Geometry check sheet. Reference: the model listing, model coordinates, mm. A direction names the side the tool comes from. Round coordinates to 2 decimals unless told otherwise and drop trailing zeros. Order: outer loops, then holes, each group sorted by start corner. A loop starts at its lowest first (then second) coordinate and runs counter-clockwise, first axis right, second up. Notation, with made-up numbers: (66.5, 88) - (123.5, 88) arc R15 ccw to (123.5, 102) - close; hole circle Ø4 at (41, 20.5). An arc over 180 degrees is marked (long way). Use a Markdown table: item, result. Add a question column.
(1) Thickness scan on line 1 along Y through (x, z) = (38.1, 0.6) (3 decimals); line 2 along Y through (x, z) = (19.05, 2); line 3 along X through (y, z) = (11.5, 1) (3 decimals). Record the ranges inside material, lowest first. Write a range as [from, to].
(2) Section check C-C on x = 38.1. Record the boundary of the cut face in (y, z) (3 decimals), then the cut area to 3 significant figures.
(3) Access from +Z, -Z, +X, -X, +Y, -Y to the whole of each face (thin tool, end or side, straight path). Record for faces 4 (the face through (-37, 11, 2.381)), 5 (the face through (-32.84, 12.03, 3.22)), 6 (the face through (-0.15, 12.39, 3.22)).
(4) Gauge pin test, flat end, axial feed: P1, Ø1, axis at x = -25.5, z = 5.5, coming from the +Y side. Record the tip position at first contact, or that the pin passes through.
(5) Mould release check, pull along X, two halves, no side actions. Record for faces 1 (the face through (34, 16.9, 3.2)), 2 (the face through (39, 11, 2.381)), 3 (the face through (20, 19.05, 3)): released by +X, released by -X, zero draft, split by the parting line, or undercut.
(6) Section check B-B on z = 1.5. Give the number of separate pieces and of enclosed holes in the cut face, then the cut area to 3 significant figures.
(7) Section check D-D on x = -38.1. Record the boundary of the cut face in (y, z), then the cut area to 3 significant figures.
(8) Section check A-A on x = 19.05. Record the boundary of the cut face in (y, z), then the cut area to 3 significant figures.
```python
from build123d import *

# Parameters (mm, degrees)
SKETCH1_W          = 88.9
SKETCH1_H          = 19.05
BASE_EXTRUDE_DEPTH = 6.35
CUT_EXTRUDE1_DEPTH = 49.775275499
CUT_EXTRUDE2_DEPTH = 49.775275499
CUT_EXTRUDE3_DEPTH = 49.775275499
CUT_EXTRUDE4_DEPTH = 49.775275499
CUT_EXTRUDE5_DEPTH = 49.775275499
FILLET1_R          = 3.175
HOLE1_D            = 7.14375
HOLE1_CBORE_D      = 10.31875
HOLE1_CBORE_DEPTH  = 3.96875
LPATTERN1_COUNT    = 2
LPATTERN1_PITCH    = 76.2
HOLE2_OUTLINE_R    = 1.5875
HOLE2_DEPTH        = 6.35
HOLE3_OUTLINE_R    = 1.5875
HOLE3_DEPTH        = 6.35
LPATTERN2_COUNT    = 2
LPATTERN2_PITCH    = 57.15


# Read off the part's stored shape, not the designer's step: Hole2, Hole3
with BuildPart() as part:
    # Sketch1 → Base-Extrude (new body)
    with BuildSketch(Plane.XY):
        with Locations((0, 9.525)):
            Rectangle(SKETCH1_W, SKETCH1_H)
    extrude(amount=BASE_EXTRUDE_DEPTH)

    # Sketch2 → Cut-Extrude1 (cut, through all)
    with BuildSketch(Plane.XY.offset(6.35)):
        Polygon((44.45, 14.2875), (25.4, 19.05), (44.45, 19.05), align=None)
    extrude(amount=-CUT_EXTRUDE1_DEPTH, mode=Mode.SUBTRACT)

    # Sketch3 → Cut-Extrude2 (cut, through all)
    with BuildSketch(Plane.XY.offset(6.35)):
        with BuildLine():
            Line((-136.365872597, 74.873193339), (-14.549677831, 19.05))
            ThreePointArc((-14.549677831, 19.05), (0, 15.875), (14.549677831, 19.05))
            Line((14.549677831, 19.05), (136.365872597, 74.873193339))
            Line((136.365872597, 74.873193339), (136.365872597, 342.868821823))
            Line((136.365872597, 342.868821823), (-136.365872597, 342.868821823))
            Line((-136.365872597, 342.868821823), (-136.365872597, 74.873193339))
        make_face()
    extrude(amount=-CUT_EXTRUDE2_DEPTH, mode=Mode.SUBTRACT)

    # Sketch4 → Cut-Extrude3 (cut, through all)
    with BuildSketch(Plane.XY.offset(6.35)):
        Polygon((-231.275885049, -20.742353447), (-44.45, 14.2875), (-19.05, 19.05), (167.775885049, 54.079853447), (97.716178156, 427.731623544), (-301.335591942, 352.909416651), align=None)
    extrude(amount=-CUT_EXTRUDE3_DEPTH, mode=Mode.SUBTRACT)

    # Sketch5 → Cut-Extrude4 (cut, through all)
    with BuildSketch(Plane.XY.offset(6.35)):
        Polygon((-36.984386732, 15.687302488), (-28.575, 8.262261056), (-28.575, 17.2640625), align=None)
    extrude(amount=-CUT_EXTRUDE4_DEPTH, mode=Mode.SUBTRACT)

    # Sketch6 → Cut-Extrude5 (cut, through all)
    with BuildSketch(Plane.XY.offset(6.35)):
        with BuildLine():
            ThreePointArc((-10.587110246, 13.878358811), (0, 12.3904375), (10.587110246, 13.878358811))
            ThreePointArc((10.587110246, 13.878358811), (14.75971189, 11.565447951), (12.446801031, 7.392846306))
            ThreePointArc((12.446801031, 7.392846306), (0, 5.6435625), (-12.446801031, 7.392846306))
            ThreePointArc((-12.446801031, 7.392846306), (-14.75971189, 11.565447951), (-10.587110246, 13.878358811))
        make_face()
    extrude(amount=-CUT_EXTRUDE5_DEPTH, mode=Mode.SUBTRACT)

    # Fillet1
    fillet1_edges = [part.edges().sort_by_distance(p)[0] for p in [
        (44.45, 14.2875, 3.175),
        (25.4, 19.05, 3.175),
        (-19.05, 19.05, 3.175),
        (-44.45, 14.2875, 3.175),
    ]]
    fillet(fillet1_edges, radius=FILLET1_R)

    # Hole1 (through all)
    with Locations(Plane.XY.offset(6.35)):
        with Locations((38.1, 7.14375)):
            hole1 = CounterBoreHole(HOLE1_D / 2, HOLE1_CBORE_D / 2, HOLE1_CBORE_DEPTH)

    # LPattern1: Hole1 ×2
    with Locations(*[(-i * LPATTERN1_PITCH, 0, 0) for i in range(1, LPATTERN1_COUNT)]):
        add(hole1, mode=Mode.SUBTRACT)

    # Hole2 outline → Hole2 (cut)
    with BuildSketch(Plane.XY):
        with Locations((28.575, 4.7625)):
            Circle(HOLE2_OUTLINE_R)
    hole2 = extrude(amount=HOLE2_DEPTH, mode=Mode.SUBTRACT)

    # Hole3 outline → Hole3 (cut)
    with BuildSketch(Plane.XY):
        with Locations((19.05, 3.175)):
            Circle(HOLE3_OUTLINE_R)
    extrude(amount=HOLE3_DEPTH, mode=Mode.SUBTRACT)

    # LPattern2: Hole2 ×2
    with Locations(*[(-i * LPATTERN2_PITCH, 0, 0) for i in range(1, LPATTERN2_COUNT)]):
        add(hole2, mode=Mode.SUBTRACT)


solid = part.part
```
Check sheet entries:
| question | item | result |
|---|---|---|
| 1 | line 1 | y = [0, 3.572], [10.716, 15.875] |
| 1 | line 2 | y = [0, 1.59], [4.76, 19.05] |
| 1 | line 3 | x = [-44.45, -32.242], [-28.575, -14.778], [14.778, 44.45] |
| 2 | outline | (0, 0) - (3.572, 0) - (3.572, 2.381) - (1.984, 2.381) - (1.984, 6.35) - (0, 6.35) - close; (10.716, 0) - (15.875, 0) - (15.875, 6.35) - (12.303, 6.35) - (12.303, 2.381) - (10.716, 2.381) - close |
| 2 | area | 42.8 mm2 |
| 3 | face 4 | +Z |
| 3 | face 5 | +Z, -Z, +Y |
| 3 | face 6 | +Z, -Z |
| 4 | P1 | stops at y = 17.93 |
| 5 | face 1 | released by +X |
| 5 | face 2 | undercut |
| 5 | face 3 | zero draft |
| 6 | separate pieces | 1 |
| 6 | enclosed holes | 6 |
| 6 | area | 1,190 mm2 |
| 7 | outline | (0, 0) - (3.57, 0) - (3.57, 2.38) - (1.98, 2.38) - (1.98, 6.35) - (0, 6.35) - close; (10.72, 0) - (15.48, 0) - (15.48, 6.35) - (12.3, 6.35) - (12.3, 2.38) - (10.72, 2.38) - close |
| 7 | area | 40.3 mm2 |
| 8 | outline | (0, 0) - (1.59, 0) - (1.59, 6.35) - (0, 6.35) - close; (4.76, 0) - (19.05, 0) - (19.05, 6.35) - (4.76, 6.35) - close |
| 8 | area | 101 mm2 |
